Could you check a few things on this model? Use its own coordinates, in mm. A direction names the side the tool comes from. Coordinates: 2 decimals unless noted, no trailing zeros. Loops run counter-clockwise (first coordinate to the right, second up) from the corner with the lowest first, then second, coordinate; pieces in that order, holes last.
1) Will these pins go through, and if not, where does the flat tip stop? P1, Ø1.8, axis at x = 45.52, y = 37.27, coming from the +Z side; P2, Ø14, axis at x = 31.5, y = 24, coming from the -Z side; P3, Ø4.5, axis at x = 41.06, y = 11.85, coming from the +Z side; P4, Ø3, axis at x = 26.5, y = 7, coming from the +Z side.
2) Imagine slicing it at A-A on x = 39.5. Please give me the cut outline in (y, z).
3) For faces 5 (the face through (30.96, 9.37, -0.74)), 6 (the face through (37.81, 12, 2.26)), 7 (the face through (34.89, 4.88, 1.48)), which set-ups out of +Z, -Z, +X, -X, +Y, -Y let a thin tool reach every point of the face, with its end or its side?
4) If I drill on line 1 along Z through (x, y) = (31.75, 37); line 2 along Y through (x, z) = (27.75, 2.55); line 3 along X through (y, z) = (36, 0.25), over which ranges is the centre line in solid material (lowest first)?
5) Thinking about a two-plate mould opening in X: for faces 1 (the face through (26.44, 8.41, -0.44)), 2 (the face through (48.432, 24, 1)), 3 (the face through (20.315, 20, 1)), 4 (the face through (43, 10, 1.5)), which applies, released by +X, released by -X, zero draft, split by the parting line, or undercut?
6) Imagine slicing it at B-B on z = 2.6. Please give me the cut outline in (x, y).
7) Imagine slicing it at C-C on y = 6. Please give me the cut outline in (x, z).
Autodesk Inventor part; units mm, degrees
ref_plane "YZ Plane" through (0, 0, 0) normal (1, 0, 0) x (0, 1, 0)
ref_plane "XZ Plane" through (0, 0, 0) normal (0, 1, 0) x (-1, 0, 0)
ref_plane "XY Plane" through (0, 0, 0) normal (0, 0, 1) x (1, 0, 0)
sketch "Sketch1" plane through (0, 0, 0) normal (0, 0, 1) x (1, 0, 0)
  line L0 (0, 61.5875) -> (62, 61.5875) construction
  line L1 (62, 61.5875) -> (62, -0.4125) construction
  line L2 (62, -0.4125) -> (0, -0.4125) construction
  line L3 (0, -0.4125) -> (0, 61.5875) construction
  line L4 (48.4322, 11.2012) -> (48.4322, 37.9079)
  line L5 (20.3147, 37.9079) -> (20.3147, 2.4417)
  line L6 (24.0433, 39.9079) -> (22.3147, 39.9079)
  line L7 (46.4322, 39.9079) -> (24.0433, 39.9079)
  arc A0 (22.3147, 39.9079) -> (20.3147, 37.9079) centre (22.3147, 37.9079) ccw
  circle A1 centre (23.179, 26.4983) radius 1.5
  circle A2 centre (45.5157, 37.2749) radius 1.5
  line L8 (16.613, -7.1773) -> (55.7088, 13.6823)
  line L9 (22.9974, 0.5619) -> (47.1149, 9.3214)
  arc A3 (20.3147, 2.4417) -> (22.9974, 0.5619) centre (22.3147, 2.4417) ccw
  arc A4 (47.1149, 9.3214) -> (48.4322, 11.2012) centre (46.4322, 11.2012) ccw
  arc A5 (48.4322, 37.9079) -> (46.4322, 39.9079) centre (46.4322, 37.9079) ccw
  point P0 (0, 0)
  point P1 (48.4322, 39.9079)
  point P2 (48.4322, 9.7998)
  point P3 (20.3147, -0.4125)
  dimension "d9" = 62
  dimension "d18" = 2
  dimension "d19" = 3
  dimension "d20" = 3
  dimension "d27" = 28.1175
  dimension "d47" = 2
extrude "Extrusion2" add sketch "Sketch1" along normal blind 3
sketch "Sketch3" plane through (0, 0, 0) normal (0, 0, -1) x (-1, 0, 0)
  circle A0 centre (-41.0584, 11.8538) radius 4
  circle A1 centre (-27.789, 6.9341) radius 4
  point P0 (0, 0)
  dimension "d51" = 8
  dimension "d52" = 8
extrude "Extrusion4" add sketch "Sketch3" along normal blind 1.5
sketch "Sketch4" plane through (0, 0, 3) normal (0, 0, 1) x (1, 0, 0)
  circle A0 centre (27.789, 6.9341) radius 4
  circle A1 centre (41.0584, 11.8538) radius 4
  circle A2 centre (41.0584, 11.8538) radius 3.25
  circle A3 centre (27.789, 6.9341) radius 3.25
  point P0 (0, 0)
  dimension "d55" = 6.5
  dimension "d56" = 6.5
extrude "Extrusion5" cut sketch "Sketch4" against normal blind 1.5 contours A2 | A3
sketch "Sketch5" plane through (41.0584, 11.8538, 1.5) normal (0, 0, 1) x (1, 0, 0)
  circle A0 centre (-13.2694, -4.9197) radius 3.25
  circle A1 centre (0, 0) radius 3.25
  point P0 (-41.0584, -11.8538)
hole "Hole1" at (27.789, 6.9341, 1.5) at (41.0584, 11.8538, 1.5) direction (0, 0, -1) diameter 4 depth 3 tip angle 118 counterbore diameter 5 counterbore depth 0.85
properties part number "bump_switch_mount"
Filled in:
1. P1: passes through
1. P2: stops at z = 0
1. P3: stops at z = 0.65
1. P4: stops at z = 1.5
2. outline: (6.56, 0) - (8.17, 0) - (8.17, -1.5) - (10.6, -1.5) - (10.6, 0.65) - (9.9, 0.65) - (9.9, 1.5) - (9, 1.5) - (9, 3) - (6.56, 3) - close; (13.11, -1.5) - (15.54, -1.5) - (15.54, 0) - (39.91, 0) - (39.91, 3) - (14.71, 3) - (14.71, 1.5) - (13.81, 1.5) - (13.81, 0.65) - (13.11, 0.65) - close
3. face 5: -Z
3. face 6: +Z
3. face 7: +Z, -Z, +X, -Y
4. line 1: z = 0 to 3
4. line 2: y = 2.29 to 3.68, 10.18 to 39.91
4. line 3: x = 20.31 to 44.73, 46.31 to 48.43
5. face 1: undercut
5. face 2: released by +X
5. face 3: released by -X
5. face 4: undercut
6. outline: (20.31, 2.44) arc R2 ccw to (23, 0.56) - (47.11, 9.32) arc R2 ccw to (48.43, 11.2) - (48.43, 37.91) arc R2 ccw to (46.43, 39.91) - (22.31, 39.91) arc R2 ccw to (20.31, 37.91) - close; hole circle Ø3 at (23.18, 26.5); hole circle Ø6.5 at (27.79, 6.93); hole circle Ø6.5 at (41.06, 11.85); hole circle Ø3 at (45.52, 37.27)
7. outline: (20.31, 0) - (23.9, 0) - (23.9, -1.5) - (26.02, -1.5) - (26.02, 0.65) - (25.47, 0.65) - (25.47, 1.5) - (24.68, 1.5) - (24.68, 3) - (20.31, 3) - close; (29.56, -1.5) - (31.68, -1.5) - (31.68, 0) - (37.97, 0) - (37.97, 3) - (30.9, 3) - (30.9, 1.5) - (30.11, 1.5) - (30.11, 0.65) - (29.56, 0.65) - close
